```python
from build123d import *

# Parameters (mm, degrees)
F1_DEPTH = 30.226
F3_DEPTH = 17.018
F5_DEPTH = 25.654
F7_DEPTH = 10.922
F9_DEPTH = 10.922
F11_D    = 25.4


with BuildPart() as f1:
    # F0 (on Top) → F1 (new body)
    with BuildSketch(Plane.XY):
        Polygon((-27.542058, -29.474055), (-13.702727, -29.474055), (72.541967, -29.474055), (116.490424, 0), (72.541967, 21.806085), (-27.542058, 21.806085), (-27.542058, 42.54153), (-78.533083, 42.54153), (-78.533083, 21.806085), (-61.017197, 21.806085), (-53.670939, 21.806085), (-53.670939, -29.474055), (-78.533083, -29.474055), (-78.533083, -50.979555), (-27.542058, -50.979555), align=None)
    extrude(amount=F1_DEPTH)

    # F2 (on face) → F3 (join)
    with BuildSketch(Plane.XY.offset(30.226)):
        Polygon((84.1086, -21.716887), (84.1086, 16.067022), (72.541967, 21.806085), (-27.542058, 21.806085), (-27.542058, -29.474055), (72.541967, -29.474055), align=None)
    extrude(amount=F3_DEPTH)

    # F4 (on face) → F5 (join)
    with BuildSketch(Plane.XY.offset(30.226)):
        Polygon((-27.542058, 42.54153), (-78.533083, 42.54153), (-78.533083, 21.806085), (-53.670939, 21.806085), (-53.670939, -29.474055), (-78.533083, -29.474055), (-78.533083, -50.979555), (-27.542058, -50.979555), align=None)
    extrude(amount=F5_DEPTH)

    # F6 (on face) → F7 (join)
    with BuildSketch(Plane.XY.offset(55.88)):
        Polygon((-53.670939, 21.806085), (-53.670939, 15.110248), (-27.542058, 15.110248), (-27.542058, 42.54153), (-78.533083, 42.54153), (-78.533083, 21.806085), align=None)
    extrude(amount=F7_DEPTH)

    # F8 (on face) → F9 (join)
    with BuildSketch(Plane.XY.offset(55.88)):
        Polygon((-53.670939, -22.706658), (-53.670939, -29.474055), (-78.533083, -29.474055), (-78.533083, -50.979555), (-27.542058, -50.979555), (-27.542058, -22.706658), align=None)
    extrude(amount=F9_DEPTH)

    # F11 (through all)
    with Locations(Plane.XZ.offset(29.474055)):
        with Locations((22.720842, 25.850486)):
            Hole(F11_D / 2)


solid = f1.part
```
The listing builds one solid part. Answer for the finished solid, in the listing's coordinates (mm). A direction names the side the tool comes from. Coordinates: 2 decimals unless noted, no trailing zeros. Order: outer loops, then holes, each group sorted by start corner. A loop starts at its lowest first (then second) coordinate and runs counter-clockwise, first axis right, second up. Notation, with made-up numbers: M 9,-11.5 L 37,-11.5 A19 ccw 37,13.5 Z; hole C 50,77.25 d7. An arc over 180 degrees is marked long. Answer as a JSON object with one key per item and string values. Group by question number.
1. Section C-C on x = -41.5 is taken. Write down the section's boundary in (y, z).
2. Flat-ended cylindrical pins translate along their axes: P1, Ø16, axis at x = 96, y = -2, coming from the +Z side; P2, Ø8, axis at x = 8.5, z = 18.5, coming from the -Y side; P3, Ø18.5, axis at y = 1.5, z = 41.5, coming from the +X side. Find the tip coordinate at first contact, or state that the pin passes through.
3. Section A-A on x = 32.5 is taken. Write down the section's boundary in (y, z).
4. Section D-D on z = 54 is taken. Write down the section's boundary in (x, y), then the cut area to 3 significant figures.
5. Straight lines are drawn through the part: line 1 (Y direction, x = -68, z = 18.5); line 2 (X direction, y = 37.5, z = 28); line 3 (Y direction, x = 31, z = 11). For each, find the intervals that lie inside material, in ascending order.
6. Determine the mould class of faces 1 (the flat face through (-53, 29, 66.802)), 2 (the flat face through (-53.671, -3, 33)), 3 (the flat face through (-53, -50.98, 33)) for opening direction Y: released by +Y, released by -Y, zero draft, split by the parting line, or undercut.
7. A tool of negligible diameter and unlimited length cuts with its end or side. For faces 4 (the flat face through (-66, 21.806, 33)), 5 (the flat face through (-41, -4, 55.88)), 6 (the flat face through (23, 21.806, 13)), 7 (the flat face through (84.109, -3, 39)), from which of +Z, -Z, +X, -X, +Y, -Y can it reach the whole face along a straight path? Write none if from no direction.
8. Section B-B on y = 13 is taken. Write down the section's boundary in (x, z).
Values follow:
{
 "1": {"outline": "M -50.98,0 L 42.54,0 L 42.54,66.8 L 15.11,66.8 L 15.11,55.88 L -22.71,55.88 L -22.71,66.8 L -50.98,66.8 Z"},
 "2": {"P1": "z = 30.23", "P2": "y = -29.47", "P3": "x = 84.11"},
 "3": {"outline": "M -29.47,0 L 21.81,0 L 21.81,17.75 L -29.47,17.75 Z; M -29.47,33.95 L 21.81,33.95 L 21.81,47.24 L -29.47,47.24 Z"},
 "4": {"outline": "M -78.53,-50.98 L -27.54,-50.98 L -27.54,42.54 L -78.53,42.54 L -78.53,21.81 L -53.67,21.81 L -53.67,-29.47 L -78.53,-29.47 Z", "area": "3,490 mm2"},
 "5": {"line 1": "-50.98 to -29.47, 21.81 to 42.54", "line 2": "-78.53 to -27.54", "line 3": "-29.47 to 21.81"},
 "6": {"face 1": "zero draft", "face 2": "undercut", "face 3": "released by -Y"},
 "7": {"face 4": "+Z, -Z, -X", "face 5": "+Z, +X, -X", "face 6": "+Z, -Z, +X, +Y", "face 7": "+Z, +X, +Y, -Y"},
 "8": {"outline": "M -53.67,0 L 90.29,0 L 90.29,30.23 L 84.11,30.23 L 84.11,47.24 L -27.54,47.24 L -27.54,55.88 L -53.67,55.88 Z; hole C 22.72,25.85 d25.4"}
}
